CAD build for the part. Positions are in the model's coordinates, mm. A direction names the side the tool comes from. Round coordinates to 2 decimals unless told otherwise and drop trailing zeros. Write each loop counter-clockwise with the first axis right and the second up, starting at its lowest first coordinate (ties: lowest second). Pieces come first, ordered by that corner, then holes. Notation, with made-up numbers: (70.5, 74) - (86.5, 74) arc R30 cw to (86.5, 105) - close; hole circle Ø2 at (86.5, 45.5). An arc over 180 degrees is marked (long way). Put each result on its own line as item: value. Start each with the question number.
Item 1: Cut at B-B (z = -12.5). Give the cut face in (x, y).
Item 2: Mould opens along Z. For faces 4 (the flat face through (4, -25, 0)), 5 (the flat face through (3, 0, -30)), 6 (the flat face through (5, -44, -43.75)) say: released by +Z, released by -Z, zero draft, split by the parting line, or undercut.
Item 3: Drill centre lines: line 1 (Z direction, x = 4, y = -10); line 2 (Z direction, x = 5, y = -48); line 3 (X direction, y = -53, z = -48). Where is each one in solid material? Low to high. Write a range as from..to.
Item 4: Cut at A-A (y = -45.5). Give the cut face in (x, z).
Item 5: Cut at D-D (z = -42). Give the cut face in (x, y).
Item 6: Pin check, flat tips, straight feed: pin 1 Ø6 at (y, z) = (-33.5, -7.5) entering from -X; pin 2 Ø0.8 at (x, z) = (2, -18.5) entering from -Y; pin 3 Ø4 at (y, z) = (-10, -47.5) entering from +X. Stop position of each tip, or through.
Item 7: Cut at C-C (x = 3.5). Give the cut face in (y, z), and give its area (3 significant figures).
Item 8: 3-axis set-ups, long thin cutter, end or side, ignore diameter. For faces 1 (the flat face through (1, -20, -30)), 2 (the flat face through (4, -26, -60)), 3 (the flat face through (5, -44, -8.75)): which of +Z, -Z, +X, -X, +Y, -Y reach the whole face in a straight line?
Autodesk Inventor part; units mm, degrees
ref_plane "YZ Plane" through (0, 0, 0) normal (1, 0, 0) x (0, 1, 0)
ref_plane "XZ Plane" through (0, 0, 0) normal (0, 1, 0) x (-1, 0, 0)
ref_plane "XY Plane" through (0, 0, 0) normal (0, 0, 1) x (1, 0, 0)
sketch "Sketch1" plane through (0, 0, 0) normal (1, 0, 0) x (0, 1, 0)
  line L0 (0, 0) -> (-65, 0)
  line L1 (-65, 0) -> (-65, -60)
  line L2 (-65, -60) -> (0, -60)
  line L3 (0, -60) -> (0, 0)
  line L4 (-40.75, -8.75) -> (-48.25, -8.75)
  line L5 (-48.25, -8.75) -> (-48.25, -16.25)
  line L6 (-48.25, -16.25) -> (-40.75, -16.25)
  line L7 (-40.75, -16.25) -> (-40.75, -8.75)
  arc A0 (-40.75, -16.25) -> (-40.75, -8.75) centre (-40.75, -12.5) ccw
  arc A1 (-48.25, -8.75) -> (-48.25, -16.25) centre (-48.25, -12.5) ccw
  line L8 (-40.75, -43.75) -> (-48.25, -43.75)
  line L9 (-48.25, -43.75) -> (-48.25, -51.25)
  line L10 (-48.25, -51.25) -> (-40.75, -51.25)
  line L11 (-40.75, -51.25) -> (-40.75, -43.75)
  arc A2 (-40.75, -51.25) -> (-40.75, -43.75) centre (-40.75, -47.5) ccw
  arc A3 (-48.25, -43.75) -> (-48.25, -51.25) centre (-48.25, -47.5) ccw
  circle A4 centre (-10, -12.5) radius 3.25
  circle A5 centre (-10, -47.5) radius 3.25
  line L12 (-20, 0) -> (-65, 0)
  line L13 (-65, 0) -> (-65, -60)
  line L14 (-65, -60) -> (-20, -60)
  line L15 (-20, -60) -> (-20, 0)
  point P0 (-20, -60)
  dimension "d1" = 60
  dimension "d4" = 7.5
  dimension "d5" = 7.5
  dimension "d8" = 8.75
  dimension "d10" = 35
  dimension "d15" = 10
  dimension "d16" = 6.5
  dimension "d17" = 6.5
  dimension "d18" = 30.75
  dimension "d19" = 65
  dimension "d20" = 7.5
  dimension "d21" = 20
extrude "Extrusion1" add sketch "Sketch1" along normal blind 6.35
extrude "Extrusion2" cut sketch "Sketch1" along normal blind 2.75 contours L15 L2 L1 L0
equation "\"d5\" = d4"
equation "\"d8\" = -0.5 * d4 + 0.5 * d1 - 0.5 * d10"
equation "\"d17\" = d16"
properties part number "mounting bracket 2"
Output values:
1. outline: (0, -20) - (2.75, -20) - (2.75, -37) - (6.35, -37) - (6.35, -13.25) - (0, -13.25) - close; (0, -6.75) - (6.35, -6.75) - (6.35, 0) - (0, 0) - close; (2.75, -65) - (6.35, -65) - (6.35, -52) - (2.75, -52) - close
2. face 4: released by +Z
2. face 5: zero draft
2. face 6: undercut
3. line 1: -60..-50.75, -44.25..-15.75, -9.25..0
3. line 2: -60..-51.25, -43.75..-16.25, -8.75..0
3. line 3: 2.75..6.35
4. outline: (2.75, -60) - (6.35, -60) - (6.35, -51.25) - (2.75, -51.25) - close; (2.75, -43.75) - (6.35, -43.75) - (6.35, -16.25) - (2.75, -16.25) - close; (2.75, -8.75) - (6.35, -8.75) - (6.35, 0) - (2.75, 0) - close
5. outline: (0, -20) - (2.75, -20) - (2.75, -65) - (6.35, -65) - (6.35, 0) - (0, 0) - close
6. pin 1: x = 2.75
6. pin 2: y = -20
6. pin 3: through
7. outline: (-65, -60) - (0, -60) - (0, 0) - (-65, 0) - close; hole (-48.25, -51.25) - (-40.75, -51.25) arc R3.75 ccw to (-40.75, -43.75) - (-48.25, -43.75) arc R3.75 ccw to start; hole (-48.25, -16.25) - (-40.75, -16.25) arc R3.75 ccw to (-40.75, -8.75) - (-48.25, -8.75) arc R3.75 ccw to start; hole circle Ø6.5 at (-10, -47.5); hole circle Ø6.5 at (-10, -12.5)
7. area: 3,630 mm2
8. face 1: +Z, -Z, -X, -Y
8. face 2: -Z, +X, -X, +Y, -Y
8. face 3: +X, -X
